Here's how the part is built. I have some questions about the finished solid (model axes, mm). A direction names the side the tool comes from. Round coordinates to 2 decimals unless told otherwise and drop trailing zeros. Order: outer loops, then holes, each group sorted by start corner. A loop starts at its lowest first (then second) coordinate and runs counter-clockwise, first axis right, second up.
```python
from build123d import *

# Parameters (mm, degrees)
F1_DEPTH = 239
F3_W     = 50
F3_H     = 549.955452
F4_DEPTH = 100
F6_DEPTH = 40


with BuildPart() as f1:
    # F0 (on Right) → F1 (new body)
    with BuildSketch(Plane.YZ):
        Polygon((305, -15.000245), (0.704454, -0.004757), (-3, 494.955207), (-48, 494.955207), (-55, -55.000245), (0, -55.000245), (305, -55.000245), align=None)
    extrude(amount=-F1_DEPTH)

    # F3 (on offset) → F4 (join)
    with BuildSketch(Plane.XZ.offset(103)):
        with Locations((-264, 219.977481)):
            Rectangle(F3_W, F3_H)
    extrude(amount=-F4_DEPTH)

    # F5 (on face) → F6 (cut)
    with BuildSketch(Plane(origin=(-289, 0, 0), x_dir=(0, -1, 0), z_dir=(-1, 0, 0))):
        with BuildLine():
            ThreePointArc((25.068039, 464.955207), (24.482252, 466.369421), (23.068039, 466.955207))
            Line((23.068039, 466.955207), (23.068039, 462.955207))
            ThreePointArc((23.068039, 462.955207), (24.482252, 463.540994), (25.068039, 464.955207))
        make_face()
        with BuildLine():
            ThreePointArc((86.530097, -46.76263), (85.829579, -45.242318), (84.21875, -44.787013))
            Line((84.21875, -44.787013), (84.841444, -48.738247))
            ThreePointArc((84.841444, -48.738247), (86.050409, -48.062111), (86.530097, -46.76263))
        make_face()
        with BuildLine():
            Line((84.841444, -48.738247), (84.21875, -44.787013))
            ThreePointArc((84.21875, -44.787013), (82.55448, -47.073977), (84.841444, -48.738247))
        make_face()
        with BuildLine():
            ThreePointArc((81.802246, -16.76263), (81.101728, -15.242318), (79.490899, -14.787013))
            Line((79.490899, -14.787013), (80.113594, -18.738247))
            ThreePointArc((80.113594, -18.738247), (81.322558, -18.062111), (81.802246, -16.76263))
        make_face()
        with BuildLine():
            Line((80.113594, -18.738247), (79.490899, -14.787013))
            ThreePointArc((79.490899, -14.787013), (77.826629, -17.073977), (80.113594, -18.738247))
        make_face()
        with BuildLine():
            ThreePointArc((75.498446, 23.23737), (74.797927, 24.757682), (73.187098, 25.212987))
            Line((73.187098, 25.212987), (73.809793, 21.261753))
            ThreePointArc((73.809793, 21.261753), (75.018757, 21.937889), (75.498446, 23.23737))
        make_face()
        with BuildLine():
            Line((73.809793, 21.261753), (73.187098, 25.212987))
            ThreePointArc((73.187098, 25.212987), (71.522829, 22.926023), (73.809793, 21.261753))
        make_face()
        with BuildLine():
            ThreePointArc((72.346545, 43.23737), (71.646027, 44.757682), (70.035198, 45.212987))
            Line((70.035198, 45.212987), (70.657893, 41.261753))
            ThreePointArc((70.657893, 41.261753), (71.866857, 41.937889), (72.346545, 43.23737))
        make_face()
        with BuildLine():
            Line((70.657893, 41.261753), (70.035198, 45.212987))
            ThreePointArc((70.035198, 45.212987), (68.370928, 42.926023), (70.657893, 41.261753))
        make_face()
        with BuildLine():
            ThreePointArc((66.042744, 83.23737), (65.342226, 84.757682), (63.731397, 85.212987))
            Line((63.731397, 85.212987), (64.354092, 81.261753))
            ThreePointArc((64.354092, 81.261753), (65.563056, 81.937889), (66.042744, 83.23737))
        make_face()
        with BuildLine():
            Line((64.354092, 81.261753), (63.731397, 85.212987))
            ThreePointArc((63.731397, 85.212987), (62.067127, 82.926023), (64.354092, 81.261753))
        make_face()
        with BuildLine():
            ThreePointArc((59.738943, 123.23737), (59.038425, 124.757682), (57.427596, 125.212987))
            Line((57.427596, 125.212987), (58.050291, 121.261753))
            ThreePointArc((58.050291, 121.261753), (59.259255, 121.937889), (59.738943, 123.23737))
        make_face()
        with BuildLine():
            Line((58.050291, 121.261753), (57.427596, 125.212987))
            ThreePointArc((57.427596, 125.212987), (55.763326, 122.926023), (58.050291, 121.261753))
        make_face()
        with BuildLine():
            ThreePointArc((56.587043, 143.23737), (55.886525, 144.757682), (54.275696, 145.212987))
            Line((54.275696, 145.212987), (54.89839, 141.261753))
            ThreePointArc((54.89839, 141.261753), (56.107355, 141.937889), (56.587043, 143.23737))
        make_face()
        with BuildLine():
            Line((54.89839, 141.261753), (54.275696, 145.212987))
            ThreePointArc((54.275696, 145.212987), (52.611426, 142.926023), (54.89839, 141.261753))
        make_face()
        with BuildLine():
            ThreePointArc((50.283242, 183.23737), (49.582724, 184.757682), (47.971895, 185.212987))
            Line((47.971895, 185.212987), (48.59459, 181.261753))
            ThreePointArc((48.59459, 181.261753), (49.803554, 181.937889), (50.283242, 183.23737))
        make_face()
        with BuildLine():
            Line((48.59459, 181.261753), (47.971895, 185.212987))
            ThreePointArc((47.971895, 185.212987), (46.307625, 182.926023), (48.59459, 181.261753))
        make_face()
        with BuildLine():
            ThreePointArc((43.979441, 223.23737), (43.278923, 224.757682), (41.668094, 225.212987))
            Line((41.668094, 225.212987), (42.290789, 221.261753))
            ThreePointArc((42.290789, 221.261753), (43.499753, 221.937889), (43.979441, 223.23737))
        make_face()
        with BuildLine():
            Line((42.290789, 221.261753), (41.668094, 225.212987))
            ThreePointArc((41.668094, 225.212987), (40.003824, 222.926023), (42.290789, 221.261753))
        make_face()
        with BuildLine():
            ThreePointArc((40.827541, 243.23737), (40.127023, 244.757682), (38.516193, 245.212987))
            Line((38.516193, 245.212987), (39.138888, 241.261753))
            ThreePointArc((39.138888, 241.261753), (40.347853, 241.937889), (40.827541, 243.23737))
        make_face()
        with BuildLine():
            Line((39.138888, 241.261753), (38.516193, 245.212987))
            ThreePointArc((38.516193, 245.212987), (36.851924, 242.926023), (39.138888, 241.261753))
        make_face()
        with BuildLine():
            ThreePointArc((34.52374, 283.23737), (33.823222, 284.757682), (32.212393, 285.212987))
            Line((32.212393, 285.212987), (32.835087, 281.261753))
            ThreePointArc((32.835087, 281.261753), (34.044052, 281.937889), (34.52374, 283.23737))
        make_face()
        with BuildLine():
            Line((32.835087, 281.261753), (32.212393, 285.212987))
            ThreePointArc((32.212393, 285.212987), (30.548123, 282.926023), (32.835087, 281.261753))
        make_face()
        with BuildLine():
            ThreePointArc((28.219939, 323.23737), (27.519421, 324.757682), (25.908592, 325.212987))
            Line((25.908592, 325.212987), (26.531287, 321.261753))
            ThreePointArc((26.531287, 321.261753), (27.740251, 321.937889), (28.219939, 323.23737))
        make_face()
        with BuildLine():
            Line((26.531287, 321.261753), (25.908592, 325.212987))
            ThreePointArc((25.908592, 325.212987), (24.244322, 322.926023), (26.531287, 321.261753))
        make_face()
        with BuildLine():
            ThreePointArc((25.068039, 374.955207), (24.482252, 376.369421), (23.068039, 376.955207))
            Line((23.068039, 376.955207), (23.068039, 372.955207))
            ThreePointArc((23.068039, 372.955207), (24.482252, 373.540994), (25.068039, 374.955207))
        make_face()
        with BuildLine():
            Line((23.068039, 372.955207), (23.068039, 376.955207))
            ThreePointArc((23.068039, 376.955207), (21.068039, 374.955207), (23.068039, 372.955207))
        make_face()
        with BuildLine():
            ThreePointArc((25.068039, 404.955207), (24.482252, 406.369421), (23.068039, 406.955207))
            Line((23.068039, 406.955207), (23.068039, 402.955207))
            ThreePointArc((23.068039, 402.955207), (24.482252, 403.540994), (25.068039, 404.955207))
        make_face()
        with BuildLine():
            Line((23.068039, 402.955207), (23.068039, 406.955207))
            ThreePointArc((23.068039, 406.955207), (21.068039, 404.955207), (23.068039, 402.955207))
        make_face()
        with BuildLine():
            ThreePointArc((25.068039, 434.955207), (24.482252, 436.369421), (23.068039, 436.955207))
            Line((23.068039, 436.955207), (23.068039, 432.955207))
            ThreePointArc((23.068039, 432.955207), (24.482252, 433.540994), (25.068039, 434.955207))
        make_face()
        with BuildLine():
            Line((23.068039, 432.955207), (23.068039, 436.955207))
            ThreePointArc((23.068039, 436.955207), (21.068039, 434.955207), (23.068039, 432.955207))
        make_face()
        with BuildLine():
            Line((23.068039, 462.955207), (23.068039, 466.955207))
            ThreePointArc((23.068039, 466.955207), (21.068039, 464.955207), (23.068039, 462.955207))
        make_face()
    extrude(amount=-F6_DEPTH, mode=Mode.SUBTRACT)


solid = f1.part
```
1) I'm going to push flat-ended pins straight in: pin 1 (5 mm diameter, centred on x = -203.5, y = 222.5, fed in from +Z); pin 2 (1.2 mm diameter, centred on y = -80.5, z = -17, fed in from -X); pin 3 (2 mm diameter, centred on y = -27, z = 324, fed in from -X); pin 4 (5 mm diameter, centred on x = -205.5, z = 66, fed in from -Y). Where does each tip first touch, or does it pass through?
2) If we section it at A-A (z = 427): Write out the boundary of the cut face in (x, y), plus the area to 3 significant figures.
3) For faces 4 (the flat face through (-239, 139, -23)), 5 (the flat face through (-117.827, 154.982, -7.607)), which set-ups out of +Z, -Z, +X, -X, +Y, -Y let a thin tool reach every point of the face, with its end or its side?
4) I need wall thicknesses on line 1 (Y direction, x = -240, z = -30.5); line 2 (X direction, y = -71.5, z = 104.5); line 3 (X direction, y = 111, z = -11). Which ranges of each line are inside material? Lowest first, please.
5) We'd pull the mould along Y, two halves only. Please class faces 1 (the flat face through (-264, -3, 224)), 2 (the flat face through (-239, -76, 216)), 3 (the flat face through (-264, -103, 224)): +Y half, -Y half, draft (parallel to the pull), parting line (faces both ways), or undercut.
6) If we section it at D-D (z = 305): Write out the boundary of the cut face in (x, y).
7) If we section it at C-C (y = 190.5): Write out the boundary of the cut face in (x, z).
8) If we section it at B-B (x = -141.5): Write out the boundary of the cut face in (y, z), plus the area to 3 significant figures.
Solutions:
1. pin 1: stops at z = -10.81
1. pin 2: stops at x = -249
1. pin 3: stops at x = -289
1. pin 4: stops at y = -53.49
2. outline: (-289, -103) - (-239, -103) - (-239, -48.86) - (0, -48.86) - (0, -2.49) - (-239, -2.49) - (-239, -3) - (-289, -3) - close
2. area: 16,100 mm2
3. face 4: +Z, -Z, -X, +Y
3. face 5: +Z, +X, -X, +Y
4. line 1: y = -103 to -3
4. line 2: x = -289 to -239
4. line 3: x = -239 to 0
5. face 1: +Y half
5. face 2: draft
5. face 3: -Y half
6. outline: (-289, -103) - (-239, -103) - (-239, -50.42) - (0, -50.42) - (0, -1.58) - (-239, -1.58) - (-239, -3) - (-289, -3) - close
7. outline: (-239, -55) - (0, -55) - (0, -9.36) - (-239, -9.36) - close
8. outline: (-55, -55) - (305, -55) - (305, -15) - (0.7, 0) - (-3, 494.96) - (-48, 494.96) - close
8. area: 42,200 mm2
